The model under review builds one solid part; all positions refer to its coordinate system, in mm. Round coordinates to 2 decimals unless told otherwise and drop trailing zeros. Order: outer loops, then holes, each group sorted by start corner. A loop starts at its lowest first (then second) coordinate and runs counter-clockwise, first axis right, second up.
```python
from build123d import *

# Parameters (mm, degrees)
CROQUIS1_R                   = 3
SALIENTE_EXTRUIR1_DEPTH      = 18
SALIENTE_EXTRUIR2_DEPTH      = 21.5
SALIENTE_EXTRUIR2_DEPTH_BACK = 1.5
CROQUIS1_2_R                 = 3
CROQUIS3_R                   = 3
CORTAR_EXTRUIR1_DEPTH        = 4.5
CROQUIS9_R                   = 1.125
SALIENTE_EXTRUIR3_DEPTH      = 55
CROQUIS10_R                  = 0.75
SALIENTE_EXTRUIR4_DEPTH      = 110


with BuildPart() as part:
    # Croquis1 → Saliente-Extruir1 (new body)
    with BuildSketch(Plane.XY):
        Circle(CROQUIS1_R)
    extrude(amount=SALIENTE_EXTRUIR1_DEPTH)

    # Croquis1<2> → Saliente-Extruir2 (add, two sides: drawn at the far end of the back side and taken through both)
    with BuildSketch(Plane.XY.offset(-SALIENTE_EXTRUIR2_DEPTH_BACK)):
        Circle(CROQUIS1_2_R)
    extrude(amount=SALIENTE_EXTRUIR2_DEPTH + SALIENTE_EXTRUIR2_DEPTH_BACK)

    # Croquis3 → Cortar-Extruir1 (cut)
    with BuildSketch(Plane(origin=(0, 0, -1.5), x_dir=(-1, 0, 0), z_dir=(0, 0, -1))):
        Circle(CROQUIS3_R)
    extrude(amount=-CORTAR_EXTRUIR1_DEPTH, mode=Mode.SUBTRACT)

    # Croquis9 → Saliente-Extruir3 (add)
    with BuildSketch(Plane.XY.offset(21.5)):
        with Locations((0, -1.15)):
            Circle(CROQUIS9_R)
        with Locations((0, 1.15)):
            Circle(CROQUIS9_R)
    extrude(amount=SALIENTE_EXTRUIR3_DEPTH)

    # Croquis10 → Saliente-Extruir4 (add)
    with BuildSketch(Plane.XY.offset(21.5)):
        with Locations((0, -1.15)):
            Circle(CROQUIS10_R)
        with Locations((0, 1.15)):
            Circle(CROQUIS10_R)
    extrude(amount=SALIENTE_EXTRUIR4_DEPTH)


solid = part.part
```
(1) Draft analysis for pull direction Y (two halves, no side actions). For faces 1 (the cylindrical face through (0.6, -0.2, 48.6)), 2 (the cylindrical face through (-3, 0, 12)), 3 (the flat face through (0, 0, 3)), state which applies: pulls with the +Y half, pulls with the -Y half, needs draft (parallel to the pull), parting line crosses it, or undercut.
Data:
face 1: undercut
face 2: parting line crosses it
face 3: needs draft
(2) To check wall thickness, follow probe 1 along Z at (x, y) = (0.3, 1.95); probe 2 along Z at (x, y) = (1.8, -1.9); probe 3 along Y at (x, z) = (0.15, 114.5). State the ranges of each line that lie inside material, in increasing order.
Data:
probe 1: z = 3 to 76.5
probe 2: z = 3 to 21.5
probe 3: y = -1.88 to -0.42, 0.42 to 1.88
(3) Insertion check: pin 1 (1.5 mm diameter, centred on x = -1, z = 24, fed in from -Y); pin 2 (1 mm diameter, centred on x = 0.5, z = 55, fed in from +Y) (3 decimals). Each pin has a flat end and moves straight along its axis. Give the tip position at first contact, or say it passes through.
Data:
pin 1: stops at y = -2.25
pin 2: stops at y = 2.275
(4) Consider section B-B (z = 105). Write out the cut boundary in (x, y).
Data:
outline: circle Ø1.5 at (0, -1.15); circle Ø1.5 at (0, 1.15)
(5) Consider section A-A (z = 61). Write out the cut boundary in (x, y) (3 decimals).
Data:
outline: circle Ø2.25 at (0, -1.15); circle Ø2.25 at (0, 1.15)
